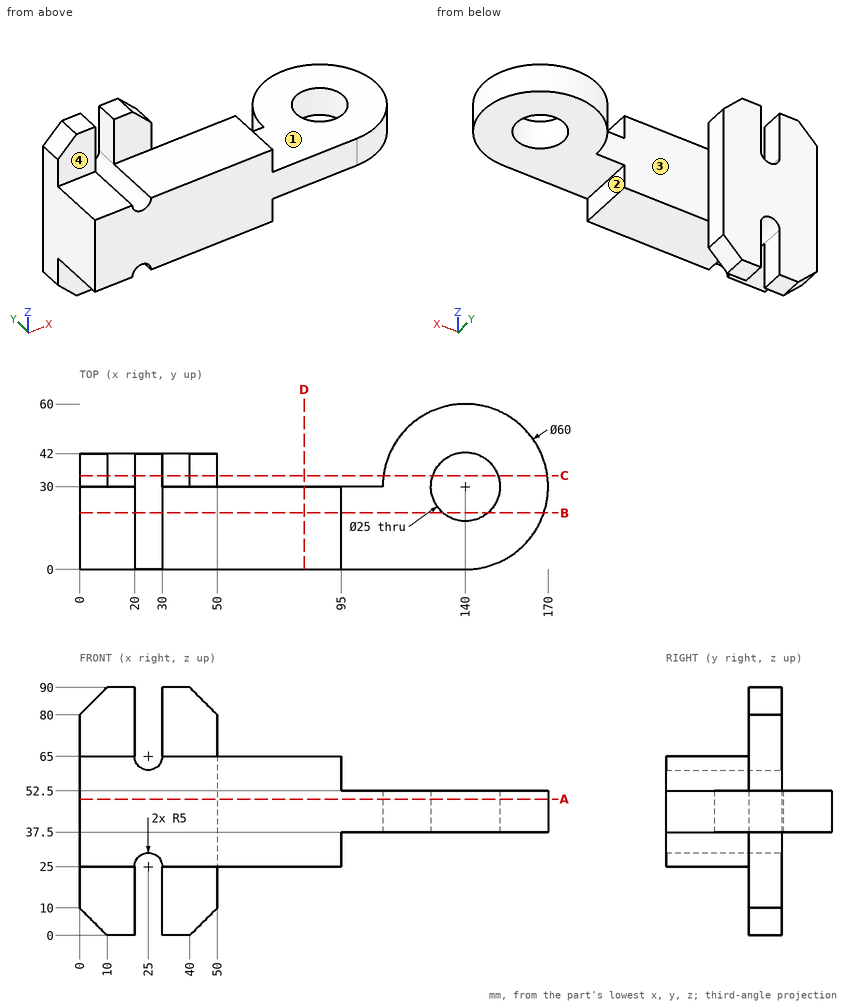
For this review, use the dimensioned drawing (mm, ordinates from the lowest corner) and the shaded views. A direction names the side the tool comes from. Coordinates: 2 decimals unless noted, no trailing zeros. Loops run counter-clockwise (first coordinate to the right, second up) from the corner with the lowest first, then second, coordinate; pieces in that order, holes last. Notation, with made-up numbers: (29, 43) - (76, 43) arc R16 cw to (76, 71) - close; hole circle Ø3 at (75.5, 83.25). An arc over 180 degrees is marked (long way). Use one line per item in the form item = value. Start each with the question number.
1) For the marked faces 1, 2, 3 and 4, list the 3-axis set-ups (+Z, -Z, +X, -X, +Y, -Y) from which the entire face can be reached by the end or side of a thin tool; tool diameter is ignored.
2) Take a section at C-C (y = 34). State the section outline as (x, z) points.
3) Take a section at B-B (y = 20.5). State the section outline as (x, z) points, plus the area to 3 significant figures.
4) Take a section at D-D (x = 81.5). State the section outline as (y, z) points, plus the area to 3 significant figures.
5) To check wall thickness, follow probe 1 along Y at (x, z) = (140, 45.25); probe 2 along X at (y, z) = (40, 39.5); probe 3 along Z at (x, y) = (68, 4.5). State the ranges of each line that lie inside material, in increasing order. Write a range as from..to.
6) For pin 1 (13 mm diameter, centred on y = 38.5, z = 35, fed in from +X); pin 2 (15 mm diameter, centred on x = 64, y = 10.5, fed in from +Z); pin 3 (18 mm diameter, centred on x = 117, y = 37.5, fed in from -Z), all flat-tipped, find the tip position at first contact; note any pin that passes through.
7) Take a section at A-A (z = 49.5). State the section outline as (x, y) points.
From the geometry:
q1.face_1 = +Z, +X, +Y, -Y
q1.face_2 = -Z, +X, +Y, -Y
q1.face_3 = +Z, -Z, +Y
q1.face_4 = +Z, +X, -X, -Y
q2.outline = (0, 10) - (10, 0) - (20, 0) - (20, 25) arc R5 cw to (30, 25) - (30, 0) - (40, 0) - (50, 10) - (50, 80) - (40, 90) - (30, 90) - (30, 65) arc R5 cw to (20, 65) - (20, 90) - (10, 90) - (0, 80) - close; (110.27, 37.5) - (128.16, 37.5) - (128.16, 52.5) - (110.27, 52.5) - close; (151.84, 37.5) - (169.73, 37.5) - (169.73, 52.5) - (151.84, 52.5) - close
q3.outline = (0, 25) - (20, 25) arc R5 cw to (30, 25) - (95, 25) - (95, 37.5) - (131.88, 37.5) - (131.88, 52.5) - (95, 52.5) - (95, 65) - (30, 65) arc R5 cw to (20, 65) - (0, 65) - close; (148.12, 37.5) - (168.46, 37.5) - (168.46, 52.5) - (148.12, 52.5) - close
q3.area = 4,580 mm2
q4.outline = (0, 25) - (30, 25) - (30, 65) - (0, 65) - close
q4.area = 1,200 mm2
q5.probe_1 = 0..17.5, 42.5..60
q5.probe_2 = 0..50, 111.72..132.5, 147.5..168.28
q5.probe_3 = 25..65
q6.pin_1 = 169.9
q6.pin_2 = 65
q6.pin_3 = 37.5
q7.outline = (0, 0) - (140, 0) arc R30 ccw (long way) to (110, 30) - (50, 30) - (50, 42) - (0, 42) - close; hole circle Ø25 at (140, 30)
